Build history of the part. All positions in model axes, mm. Face numbers are marked on the shaded views. A direction names the side the tool comes from. Give positions to 0.01 mm unless a question says otherwise; leave off trailing zeros. Write each loop counter-clockwise with the first axis right and the second up, starting at its lowest first coordinate (ties: lowest second). Pieces come first, ordered by that corner, then holes. Notation, with made-up numbers: (27.5, 33.5) - (81.5, 33.5) arc R12 ccw to (81.5, 42.5) - close; hole circle Ø11 at (26.5, -3.5). An arc over 180 degrees is marked (long way). Use one line per item in the form item = value. Start each with the question number.
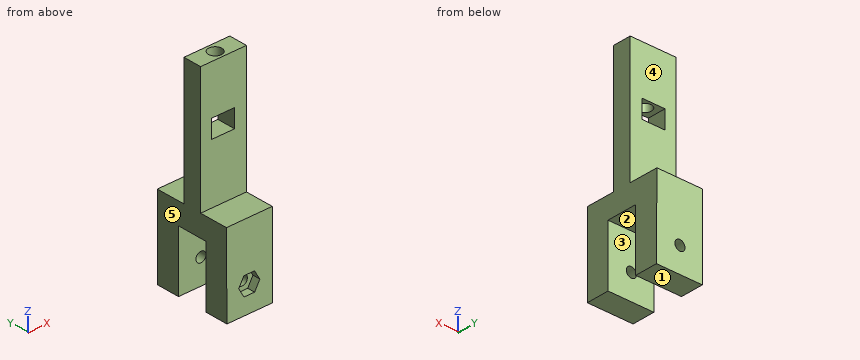
from build123d import *

# Parameters (mm, degrees)
F0_W     = 15
F0_H     = 43.4799888134
F0_W_2   = 7.5
F0_H_2   = 6
F1_DEPTH = 6
F3_DEPTH = 15
F5_D     = 4.4
F5_DEPTH = 20
F5_TIP   = 1.3218933619
F7_D     = 3.3
F7_DEPTH = 40
F7_TIP   = 0.9914200214
F8_DEPTH = 2.5


with BuildPart() as f1:
    # F0 (on Front) → F1 (new body)
    with BuildSketch(Plane.XZ):
        with Locations((0.1361690943, 49.7399944067)):
            Rectangle(F0_W, F0_H)
        with Locations((0, 52.4799888134)):
            Rectangle(F0_W_2, F0_H_2, mode=Mode.SUBTRACT)
    extrude(amount=F1_DEPTH)

    # F2 (on face) → F3 (join)
    with BuildSketch(Plane.YZ.offset(7.6361690943)):
        Polygon((9.5002116757, 3), (9.6573423812, 30), (0, 30.0562024082), (0, 28), (-6, 28), (-6, 30.0911203428), (-15.3422342746, 30.1454889303), (-15.5002116757, 3), (-8, 3), (-8, 23), (2, 23), (2, 3), align=None)
    extrude(amount=-F3_DEPTH)

    # F5
    with Locations(Plane.XY.offset(71.4799888134)):
        with Locations((0.1361690943, -3)):
            Hole(F5_D / 2, depth=F5_DEPTH)
            with Locations((0, 0, -(F5_DEPTH + F5_TIP / 2))):  # 118° drill point
                Cone(0, F5_D / 2, F5_TIP, mode=Mode.SUBTRACT)

    # F7
    with Locations(Plane(origin=(0, -15.5171451022, 0.0903044429), x_dir=(1, 0, 0), z_dir=(0, -0.9999830662, 0.0058195572))):
        with Locations((0, 11.2554198566)):
            Hole(F7_D / 2, depth=F7_DEPTH)
            with Locations((0, 0, -(F7_DEPTH + F7_TIP / 2))):  # 118° drill point
                Cone(0, F7_D / 2, F7_TIP, mode=Mode.SUBTRACT)

    # F6 (on face) → F8 (cut)
    with BuildSketch(Plane(origin=(0, -15.5171451022, 0.0903044429), x_dir=(1, 0, 0), z_dir=(0, -0.9999830662, 0.0058195572))):
        Polygon((1.7320508076, 14.2554198566), (-1.7320508076, 14.2554198566), (-3.4641016151, 11.2554198566), (-1.7320508076, 8.2554198566), (1.7320508076, 8.2554198566), (3.4641016151, 11.2554198566), align=None)
    extrude(amount=-F8_DEPTH, mode=Mode.SUBTRACT)


solid = f1.part
(1) Which spindle directions (+Z, -Z, +X, -X, +Y, -Y) get a long thin tool onto all of the face, cutting with end or side? Do the marked faces 1 and 2. Say none if no direction does.
(2) Pin check, flat tips, straight feed: pin 1 Ø3.5 at (x, y) = (0.14, -3) entering from -Z; pin 2 Ø8 at (x, y) = (2, -5.5) entering from -Z; pin 3 Ø1 at (x, z) = (-1.5, 41) entering from +Y; pin 4 Ø1 at (y, z) = (0.5, 20.5) entering from -X. Stop position of each tip, or through.
(3) Cut at A-A, the plane z = 51.5. Give the cut face in (x, y), then the cut area to 3 significant figures.
(4) Two-plate mould, pull along Y, no slides. Class the marked faces 3, 4 and 5: +Y half, -Y half, draft (parallel to the pull), parting line (faces both ways), or undercut.
(5) Cut at C-C, the plane z = 60. Give the cut face in (x, y).
(6) Cut at D-D, the plane y = -3. Give the cut face in (x, z), then the cut area to 3 significant figures.
(7) Wall check: line 1 (Y direction, x = 4, z = 15); line 2 (Y direction, x = -5.5, z = 61); line 3 (Z direction, x = -5.5, y = -4). Give the ranges that are in metal, low to high. Write a range as from..to.
(8) Cut at B-B, the plane x = 0.75. State how many separate pieces and enclosed holes the cut face has, then the cut area to 3 significant figures.
Solution:
q1.face_1 = -Z, +X, -X, +Y, -Y
q1.face_2 = -Z, +X, -X
q2.pin_1 = 23
q2.pin_2 = 3
q2.pin_3 = 0
q2.pin_4 = through
q3.outline = (-7.36, -6) - (-3.75, -6) - (-3.75, 0) - (-7.36, 0) - close; (3.75, -6) - (7.64, -6) - (7.64, 0) - (3.75, 0) - close
q3.area = 45.0 mm2
q4.face_3 = undercut
q4.face_4 = +Y half
q4.face_5 = draft
q5.outline = (-7.36, -6) - (7.64, -6) - (7.64, 0) - (-7.36, 0) - close; hole circle Ø4.4 at (0.14, -3)
q6.outline = (-7.36, 23) - (7.64, 23) - (7.64, 71.48) - (2.34, 71.48) - (2.34, 55.48) - (3.75, 55.48) - (3.75, 49.48) - (-3.75, 49.48) - (-3.75, 55.48) - (-2.06, 55.48) - (-2.06, 71.48) - (-7.36, 71.48) - close
q6.area = 612 mm2
q7.line_1 = -15.43..-8, 2..9.57
q7.line_2 = -6..0
q7.line_3 = 23..71.48
q8.separate_pieces = 5
q8.enclosed_holes = 0
q8.area = 570 mm2
